```python
from build123d import *

# Parameters (mm, degrees)
F1_DEPTH = 1.6


with BuildPart() as f1:
    # F0 (on Top) → F1 (new body, symmetric)
    with BuildSketch(Plane.XY):
        with BuildLine():
            Line((-12.2, 3.2), (-12.2, 0))
            add(Edge.make_bspline(
                [(-12.2, 0), (-9.118693519, -7.9558323076), (-6.0373870379, -15.9116646152), (-2.9560805569, -19.3)],
                knots=[0, 0, 0, 0, 0.3788491575, 0.3788491575, 0.3788491575, 0.3788491575], degree=3))
            Line((-2.9560805569, -19.3), (2.9560805569, -19.3))
            add(Edge.make_bspline(
                [(2.9560805569, -19.3), (6.0373870379, -15.9116646152), (9.118693519, -7.9558323076), (12.2, 0)],
                knots=[0.6211508425, 0.6211508425, 0.6211508425, 0.6211508425, 1, 1, 1, 1], degree=3))
            Line((12.2, 0), (6.1, 0))
            Line((6.1, 0), (6.1, 3.2))
            Line((6.1, 3.2), (0, 3.2))
            Line((0, 3.2), (0, 0))
            Line((0, 0), (-6.1, 0))
            Line((-6.1, 0), (-6.1, 3.2))
            Line((-6.1, 3.2), (-12.2, 3.2))
        make_face()
    extrude(amount=F1_DEPTH, both=True)


solid = f1.part
```
Model file for the job. Use its own axes, mm. A direction names the side the tool comes from. Give positions to 0.01 mm unless a question says otherwise; leave off trailing zeros.
1) 3-axis set-ups, long thin cutter, end or side, ignore diameter. For faces 1 (the flat face through (-6.1, 2, 0)), 2 (the flat face through (0, -19.3, 0)), 3 (the flat face through (6.1, 2, 0)): which of +Z, -Z, +X, -X, +Y, -Y reach the whole face in a straight line?
2) Wall check: probe 1 along X at (y, z) = (2, -1.3); probe 2 along Y at (x, z) = (6.75, 1.25); probe 3 along Y at (x, z) = (9.5, -0.1). Give the ranges that are in metal, low to high.
3) Pin check, flat tips, straight feed: pin 1 (1.6 mm diameter, centred on y = 1.5, z = 0, fed in from +X); pin 2 (1.6 mm diameter, centred on x = 10.5, z = -0.5, fed in from +Y). Stop position of each tip, or through.
Computed:
1. face 1: +Z, -Z, +Y
1. face 2: +Z, -Z, +X, -X, -Y
1. face 3: +Z, -Z, +X, +Y
2. probe 1: x = -12.2 to -6.1, 0 to 6.1
2. probe 2: y = -13.14 to 0
2. probe 3: y = -6.86 to 0
3. pin 1: stops at x = 6.1
3. pin 2: stops at y = 0
